The figure shows three views and two pictorial views of one solid part (mm, origin at its lowest corner). Answer the questions. A direction names the side the tool comes from. Coordinates: 2 decimals unless noted, no trailing zeros. Loops run counter-clockwise (first coordinate to the right, second up) from the corner with the lowest first, then second, coordinate; pieces in that order, holes last. Notation, with made-up numbers: (40, 40) - (54, 40) arc R22 ccw to (54, 75) - close; hole circle Ø6 at (10.5, -17). An arc over 180 degrees is marked (long way). Return JSON: item names as keys, results as strings. Group by question number.
1. Section C-C (y = 2.25) is taken. Write down the section's boundary in (x, z).
2. Find the intervals of material crossed by line 1 along Z through (x, y) = (20, 7.5); line 2 along Y through (x, z) = (11, 27.5); line 3 along Z through (x, y) = (27.5, 1.25), in increasing order.
3. Section A-A (x = 20) is taken. Write down the section's boundary in (y, z).
4. Each of these flat-tipped pins is pushed along its axis until it touches: P1, Ø5, axis at x = 35.5, y = 5.5, coming from the -Z side; P2, Ø6, axis at y = 13.5, z = 4, coming from the +X side; P3, Ø20, axis at x = 20, z = 20, coming from the -Y side. Where does it stop, or does it pass through?
5. The mould has two halves that part along Z. Classify the marked faces 3, 4 and 5: pulls with the +Z half, pulls with the -Z half, needs draft (parallel to the pull), parting line crosses it, or undercut.
6. Section B-B (y = 6) is taken. Write down the section's boundary in (x, z).
7. Which of the six approach directions +Z, -Z, +X, -X, +Y, -Y give full straight-line access (tool end or side, diameter ignored) to the marked faces 1 and 2?
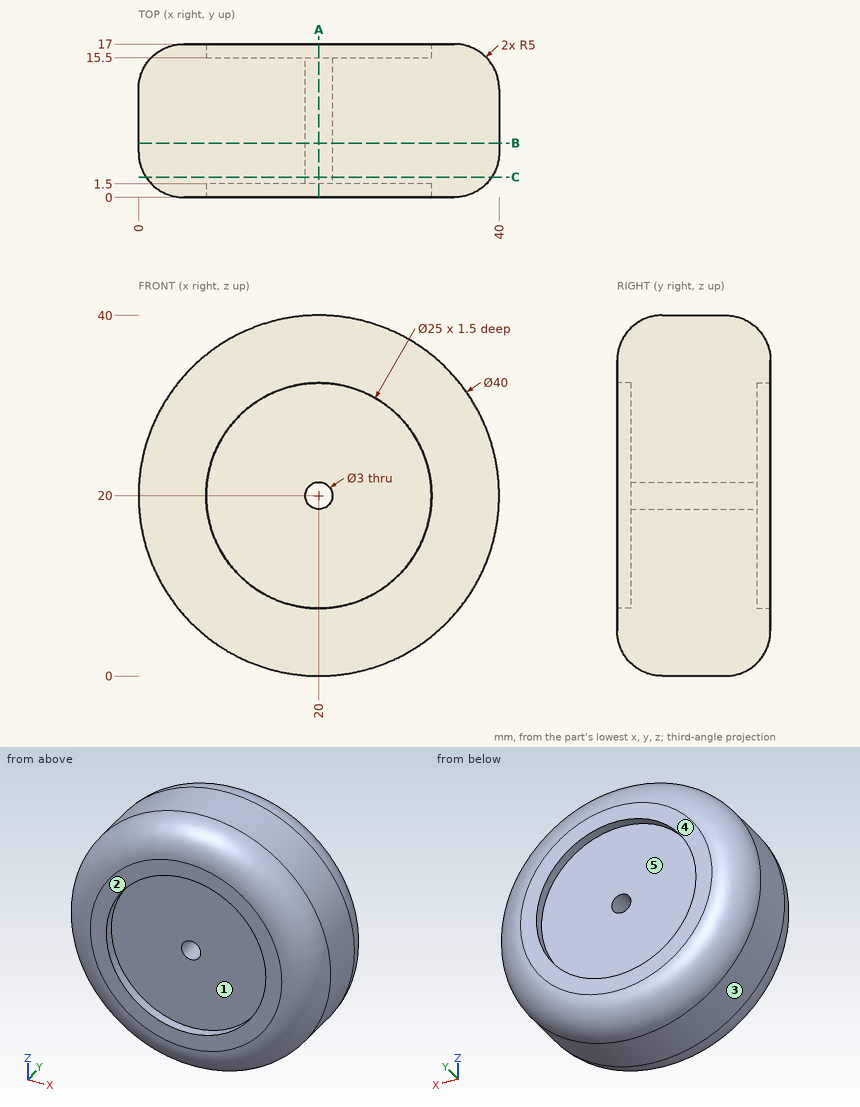
The answers:
{
 "1": {"outline": "circle Ø38.35 at (20, 20); hole circle Ø3 at (20, 20)"},
 "2": {"line 1": "z = 0 to 18.5, 21.5 to 40", "line 2": "y = 1.5 to 15.5", "line 3": "z = 3.3 to 10, 30 to 36.7"},
 "3": {"outline": "(0, 5) arc R5 ccw to (5, 0) - (12, 0) arc R5 ccw to (17, 5) - (17, 7.5) - (15.5, 7.5) - (15.5, 18.5) - (1.5, 18.5) - (1.5, 7.5) - (0, 7.5) - close; (0, 32.5) - (1.5, 32.5) - (1.5, 21.5) - (15.5, 21.5) - (15.5, 32.5) - (17, 32.5) - (17, 35) arc R5 ccw to (12, 40) - (5, 40) arc R5 ccw to (0, 35) - close"},
 "4": {"P1": "stops at z = 4.8", "P2": "stops at x = 35.04", "P3": "stops at y = 1.5"},
 "5": {"face 3": "parting line crosses it", "face 4": "needs draft", "face 5": "undercut"},
 "6": {"outline": "circle Ø40 at (20, 20); hole circle Ø3 at (20, 20)"},
 "7": {"face 1": "-Y", "face 2": "+Z, -Z, +X, -X, -Y"}
}
